Build history of the part. All positions in model axes, mm. Face numbers are marked on the shaded views. A direction names the side the tool comes from. Give positions to 0.01 mm unless a question says otherwise; leave off trailing zeros. Write each loop counter-clockwise with the first axis right and the second up, starting at its lowest first coordinate (ties: lowest second). Pieces come first, ordered by that corner, then holes. Notation, with made-up numbers: (71, 35.5) -> (106, 35.5) arc R19 cw to (106, 71.5) -> close; hole circle Ø7 at (25.5, 36). An arc over 180 degrees is marked (long way). Put each result on its own line as item: value.
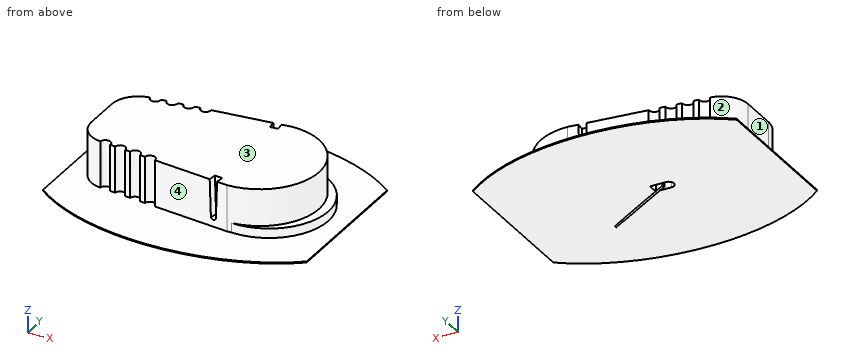
from build123d import *

# Parameters (mm, degrees)
SENSOR_HEIGHT_DEPTH               = 9
SENSOR_LIP_HEIGHT_DEPTH           = 2
SHORT_SIDE_EDGE_ROUNDING_R        = 5
PATCH_DEPTH                       = 0.2
SENSOR_HOLES_R                    = 1
EXTRUDED_SENSOR_HOLES_DEPTH       = 8.8
BOTTOM_TRIANGLE_CUT_DEPTH         = 1.5
TOP_TRIANGLE_CUT_DEPTH            = 1.5
FILAMENT_HOLE_CUT_DEPTH           = 2.5
FILAMENT_PROFILE_R                = 0.175
SENSING_START                     = -1.8
SENSING_FILAMENT_R                = 0.175
SENSING_FILAMENT_R_2              = 0.15
SENSING_PORTION_OF_FILAMENT_DEPTH = 1.8


# Read off the part's stored shape, not the designer's step: Sensor Lip Height
with BuildPart() as part:
    # Basic Sensor Dimensions → Sensor Height (new body)
    with BuildSketch(Plane.XY):
        with BuildLine():
            Line((-21.5, 8), (-21.5, -8))
            Line((-21.5, -8), (8.5, -11.25))
            ThreePointArc((8.5, -11.25), (19.75, 0), (8.5, 11.25))
            Line((8.5, 11.25), (-21.5, 8))
        make_face()
    extrude(amount=SENSOR_HEIGHT_DEPTH)

    # Sensor Lip Height outline → Sensor Lip Height (add)
    with BuildSketch(Plane.XY):
        with BuildLine():
            ThreePointArc((9.375, -11.215920604), (21.5, 0), (9.375, 11.215920604))
            ThreePointArc((9.375, 11.215920604), (19.75, 0), (9.375, -11.215920604))
        make_face()
    extrude(amount=SENSOR_LIP_HEIGHT_DEPTH)

    # Short Side Edge Rounding
    short_side_edge_rounding_edges = [part.edges().sort_by_distance(p)[0] for p in [
        (-21.5, -8, 4.5),
        (-21.5, 8, 4.5),
    ]]
    fillet(short_side_edge_rounding_edges, radius=SHORT_SIDE_EDGE_ROUNDING_R)

    # Basic Sensor Dimensions<7> → Patch (add)
    with BuildSketch(Plane.XY):
        with BuildLine():
            Line((25, 13.737877927), (25, -13.737877927))
            add(Edge.make_bspline(
                [(-25, -13.737877927), (0, -33.647845937), (25, -13.737877927)],
                knots=[3.834752561, 3.834752561, 3.834752561, 5.5900254, 5.5900254, 5.5900254], degree=2, weights=[1, 0.638971066, 1]))
            Line((-25, -13.737877927), (-25, 13.737877927))
            add(Edge.make_bspline(
                [(25, 13.737877927), (0, 33.647845937), (-25, 13.737877927)],
                knots=[0.693159908, 0.693159908, 0.693159908, 2.448432746, 2.448432746, 2.448432746], degree=2, weights=[1, 0.638971066, 1]))
        make_face()
    extrude(amount=PATCH_DEPTH)

    # Sensor Holes → Extruded Sensor Holes (cut)
    with BuildSketch(Plane.XY.offset(9)):
        with Locations((-16.044332748, -8.591030619)):
            Circle(SENSOR_HOLES_R)
        with Locations((-13.044332748, -8.916030619)):
            Circle(SENSOR_HOLES_R)
        with Locations((-10.044332748, -9.241030619)):
            Circle(SENSOR_HOLES_R)
        with Locations((-7.044332748, -9.566030619)):
            Circle(SENSOR_HOLES_R)
        with Locations((-10.044332748, 9.241030619)):
            Circle(SENSOR_HOLES_R)
        with Locations((-7.044332748, 9.566030619)):
            Circle(SENSOR_HOLES_R)
        with Locations((-13.044332748, 8.916030619)):
            Circle(SENSOR_HOLES_R)
        with Locations((-16.044332748, 8.591030619)):
            Circle(SENSOR_HOLES_R)
    extrude(amount=-EXTRUDED_SENSOR_HOLES_DEPTH, mode=Mode.SUBTRACT)

    # Bottom Triangle → Bottom Triangle Cut (cut)
    with BuildSketch(Plane(origin=(-1.106012767, -10.209348617, 0), x_dir=(0.9941830955390242, -0.10770316868339427, 0), z_dir=(-0.10770316868339427, -0.9941830955390242, 0))):
        with BuildLine():
            Line((6.91221696, 1.5), (6.91221696, 9))
            Line((6.91221696, 9), (6.16221696, 9))
            Line((6.16221696, 9), (6.41221696, 1.790726708))
            add(Edge.make_bspline(
                [(6.41221696, 1.790726708), (6.66221696, 1.5), (6.91221696, 1.5)],
                knots=[0, 0, 0, 0.5, 0.5, 0.5], degree=2))
        make_face()
        with BuildLine():
            Line((7.41221696, 1.790726708), (7.66221696, 9))
            Line((7.66221696, 9), (6.91221696, 9))
            Line((6.91221696, 9), (6.91221696, 1.5))
            add(Edge.make_bspline(
                [(6.91221696, 1.5), (7.16221696, 1.5), (7.41221696, 1.790726708)],
                knots=[0.5, 0.5, 0.5, 1, 1, 1], degree=2))
        make_face()
    extrude(amount=-BOTTOM_TRIANGLE_CUT_DEPTH, mode=Mode.SUBTRACT)

    # Top Triangle → Top Triangle Cut (cut)
    with BuildSketch(Plane(origin=(-1.106012767, 10.209348617, 0), x_dir=(0.9941830955390242, 0.10770316868339432, 0), z_dir=(-0.10770316868339432, 0.9941830955390242, 0))):
        with BuildLine():
            Line((6.91221696, -9), (7.66221696, -9))
            Line((7.66221696, -9), (7.41221696, -1.790726708))
            add(Edge.make_bspline(
                [(6.91221696, -1.5), (7.16221696, -1.5), (7.41221696, -1.790726708)],
                knots=[0.5, 0.5, 0.5, 1, 1, 1], degree=2))
            Line((6.91221696, -1.5), (6.91221696, -9))
        make_face()
        with BuildLine():
            Line((6.16221696, -9), (6.91221696, -9))
            Line((6.91221696, -9), (6.91221696, -1.5))
            add(Edge.make_bspline(
                [(6.41221696, -1.790726708), (6.66221696, -1.5), (6.91221696, -1.5)],
                knots=[0, 0, 0, 0.5, 0.5, 0.5], degree=2))
            Line((6.41221696, -1.790726708), (6.16221696, -9))
        make_face()
    extrude(amount=-TOP_TRIANGLE_CUT_DEPTH, mode=Mode.SUBTRACT)

    # Filament Hole → Filament Hole Cut (cut)
    with BuildSketch(Plane(origin=(0, 0, 0), x_dir=(-1, 0, 0), z_dir=(0, 0, -1))):
        with BuildLine():
            Line((4.5, 1), (1.5, 1))
            Line((1.5, 1), (1.5, -1))
            Line((1.5, -1), (4.5, -1))
            ThreePointArc((4.5, -1), (5.5, 0), (4.5, 1))
        make_face()
    extrude(amount=-FILAMENT_HOLE_CUT_DEPTH, mode=Mode.SUBTRACT)

    # Filament: sweep along a curve in space
    with BuildLine() as filament_path:
        Line((-3.5, 0, 0), (-3.5, 0, 2.5))
        Line((-3.5, 0, 0), (5.59326674, 0, -5.25))
    # Filament profile (on start of the path) → Filament (sweep)
    with BuildSketch(Plane(origin=(5.59326674, 0, -5.25), x_dir=(-0.500000000000001, 0, -0.866025403784438), z_dir=(-0.866025403784438, -1.4044495267806857e-15, 0.500000000000001))):
        Circle(FILAMENT_PROFILE_R)
    sweep(path=filament_path.line, transition=Transition.RIGHT)

    # Sensing Filament → Sensing Portion of Filament (cut)
    with BuildSketch(Plane(origin=(6.46826674, 0, -3.734455543), x_dir=(-0.500000000000001, 0, -0.866025403784438), z_dir=(0.866025403784438, 1.066393786355781e-15, -0.500000000000001)).offset(SENSING_START)):
        with Locations((1.75, 0)):
            Circle(SENSING_FILAMENT_R)
        with Locations((1.75, 0)):
            Circle(SENSING_FILAMENT_R_2, mode=Mode.SUBTRACT)
    extrude(amount=SENSING_PORTION_OF_FILAMENT_DEPTH, mode=Mode.SUBTRACT)


solid = part.part
1) Slice it at A-A (z = 6.5). Write the cut outline in (x, y).
Filled sheet:
outline: (-21.5, -3.51) arc R5 ccw to (-17.04, -8.48) arc R1 cw to (-15.05, -8.7) -> (-14.04, -8.81) arc R1 cw to (-12.05, -9.02) -> (-11.04, -9.13) arc R1 cw to (-9.05, -9.35) -> (-8.04, -9.46) arc R1 cw to (-6.05, -9.67) -> (5.11, -10.88) -> (5.27, -9.39) -> (6.59, -9.53) -> (6.43, -11.03) -> (8.5, -11.25) arc R11.25 ccw to (8.5, 11.25) -> (6.43, 11.03) -> (6.59, 9.53) -> (5.27, 9.39) -> (5.11, 10.88) -> (-6.05, 9.67) arc R1 cw to (-8.04, 9.46) -> (-9.05, 9.35) arc R1 cw to (-11.04, 9.13) -> (-12.05, 9.02) arc R1 cw to (-14.04, 8.81) -> (-15.05, 8.7) arc R1 cw to (-17.04, 8.48) arc R5 ccw to (-21.5, 3.51) -> close
2) Pin check, flat tips, straight feed: pin 1 (4 mm diameter, centred on x = -10, y = -2, fed in from -Z); pin 2 (3 mm diameter, centred on x = -3, z = 1.5, fed in from +Y); pin 3 (3.5 mm diameter, centred on y = -1.5, z = 6, fed in from -X). Stop position of each tip, or through.
Filled sheet:
pin 1: z = 0
pin 2: y = 21.45
pin 3: x = -21.5
3) Wall check: L1, parallel to Z at x = -14.5, y = -12.5; L2, parallel to Y at x = -9, z = 4; L3, parallel to Z at x = 4.5, y = 10. Give the ranges that are in metal, low to high.
Filled sheet:
L1: 0 to 0.2
L2: -9.35 to 9.35
L3: 0 to 9
4) Tool access for the marked faces 1, 2, 3 and 4: list every direction of +Z, -Z, +X, -X, +Y, -Y with a clear straight run to the whole face (end or side of a thin tool).
Filled sheet:
face 1: +Z, -X, +Y, -Y
face 2: +Z, -X, +Y
face 3: +Z, +X, -X, +Y, -Y
face 4: +Z, -X, -Y
